Source: CAD feature listing. Evaluate the final solid. Frame: model axes, mm. Round coordinates to 2 decimals unless told otherwise and drop trailing zeros. Loops run counter-clockwise (first coordinate to the right, second up) from the corner with the lowest first, then second, coordinate; pieces in that order, holes last.
Item 1: Section query D-D on z = 1.5. Give the number of separate pieces and of enclosed holes in the cut face, then the cut area to 3 significant figures.
Item 2: Section query B-B on x = 19.05. Return loops of the section in (y, z) (3 decimals), then the cut area to 3 significant figures.
Item 3: Ray query, L1, parallel to Y at x = 25.4, z = -0.75; L2, parallel to X at y = 88, z = 0 (3 decimals); L3, parallel to Y at x = -24.5, z = 1.75. Return the intervals inside material, ascending.
Item 4: First-contact query: P1, Ø4.5, axis at x = -0.06, y = -40.99, coming from the -Z side. Flat tip, straight axial feed; report the tip coordinate or a pass-through.
Item 5: Section query C-C on y = -57.15. Return loops of the section in (x, z) (3 decimals), then the cut area to 3 significant figures.
Item 6: Section query A-A on y = 44.45. Return loops of the section in (x, z) (3 decimals).
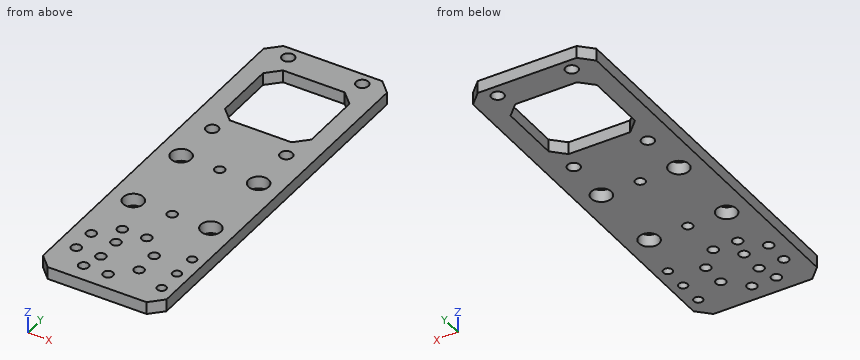
```python
from build123d import *

# Parameters (mm, degrees)
SKETCH1_W                       = 63.5
SKETCH1_H                       = 196.85
BOSS_EXTRUDE1_DEPTH             = 3.175
SKETCH2_R                       = 2.54
SKETCH2_R_2                     = 5.175
CUT_EXTRUDE1_DEPTH              = 7.35
SKETCH3_W                       = 44.45
SKETCH3_H                       = 44.45
CUT_EXTRUDE2_DEPTH              = 7.35
SKETCH4_R                       = 3.175
CUT_EXTRUDE3_DEPTH              = 7.35
CHAMFER1_SIZE                   = 6.35
SKETCH5_R                       = 2.286
CUT_EXTRUDE4_DEPTH              = 7.35
F_10_CLEARANCE_HOLE1_AT_2_COUNT = 2
F_10_CLEARANCE_HOLE1_AT_2_PITCH = 13.97
F_10_CLEARANCE_HOLE1_AT_3_COUNT = 2
F_10_CLEARANCE_HOLE1_AT_3_PITCH = 34.687510721
F_10_CLEARANCE_HOLE1_AT_4_COUNT = 2
F_10_CLEARANCE_HOLE1_AT_4_PITCH = 31.75
SKETCH9_R                       = 2.5527
CUT_EXTRUDE6_DEPTH              = 7.35


with BuildPart() as part:
    # Sketch1 → Boss-Extrude1 (new body, symmetric)
    with BuildSketch(Plane.XY):
        with Locations((0, 15.875)):
            Rectangle(SKETCH1_W, SKETCH1_H)
    extrude(amount=BOSS_EXTRUDE1_DEPTH, both=True)

    # Sketch2 → Cut-Extrude1 (cut, through all)
    with BuildSketch(Plane.XY.offset(3.175)):
        with Locations((0, 19.85)):
            Circle(SKETCH2_R)
        with Locations((0, -19.85)):
            Circle(SKETCH2_R)
        with Locations((-19.939, 19.939)):
            Circle(SKETCH2_R_2)
        with Locations((19.939, 19.939)):
            Circle(SKETCH2_R_2)
        with Locations((19.939, -19.939)):
            Circle(SKETCH2_R_2)
        with Locations((-19.939, -19.939)):
            Circle(SKETCH2_R_2)
    extrude(amount=-CUT_EXTRUDE1_DEPTH, mode=Mode.SUBTRACT)

    # Sketch3 → Cut-Extrude2 (cut, through all)
    with BuildSketch(Plane.XY.offset(3.175)):
        with Locations((0, 76.2)):
            Rectangle(SKETCH3_W, SKETCH3_H)
    extrude(amount=-CUT_EXTRUDE2_DEPTH, mode=Mode.SUBTRACT)

    # Sketch4 → Cut-Extrude3 (cut, through all)
    with BuildSketch(Plane.XY.offset(3.175)):
        with Locations((-19.05, 107.95)):
            Circle(SKETCH4_R)
        with Locations((19.05, 107.95)):
            Circle(SKETCH4_R)
        with Locations((19.05, 44.45)):
            Circle(SKETCH4_R)
        with Locations((-19.05, 44.45)):
            Circle(SKETCH4_R)
    extrude(amount=-CUT_EXTRUDE3_DEPTH, mode=Mode.SUBTRACT)

    # Chamfer1
    chamfer1_edges = [part.edges().sort_by_distance(p)[0] for p in [
        (22.225, 98.425, 0),
        (22.225, 53.975, 0),
        (-22.225, 53.975, 0),
        (-22.225, 98.425, 0),
        (31.75, -82.55, 0),
        (-31.75, -82.55, 0),
        (-31.75, 114.3, 0),
        (31.75, 114.3, 0),
    ]]
    chamfer(chamfer1_edges, length=CHAMFER1_SIZE)

    # Sketch5 → Cut-Extrude4 (cut, through all)
    with BuildSketch(Plane(origin=(0, 0, -3.175), x_dir=(-1, 0, 0), z_dir=(0, 0, -1))):
        with Locations((-25.4, -44.45)):
            Circle(SKETCH5_R)
        with Locations((-25.4, -57.15)):
            Circle(SKETCH5_R)
        with Locations((-25.4, -69.85)):
            Circle(SKETCH5_R)
    extrude(amount=-CUT_EXTRUDE4_DEPTH, mode=Mode.SUBTRACT)

    # Sketch8 → 10 Clearance Hole1 (revolve, cut)
    with BuildSketch(Plane(origin=(-22.514461018, -50.863820715, 3.175), x_dir=(0, -1, 0), z_dir=(1, 0, 0))):
        Polygon((0, 0), (0, 20.583816902), (2.5527, 19.05), (2.5527, 0), align=None)
    f_10_clearance_hole1 = revolve(axis=Axis((-22.514461018, -50.863820715, 9.525), (0, 0, -1)), mode=Mode.SUBTRACT)

    # 10 Clearance Hole1 at 2: 10 Clearance Hole1 ×2
    with Locations(*[Vector(0.707106781, 0.707106781, 0) * (i * F_10_CLEARANCE_HOLE1_AT_2_PITCH) for i in range(1, F_10_CLEARANCE_HOLE1_AT_2_COUNT)]):
        add(f_10_clearance_hole1, mode=Mode.SUBTRACT)

    # 10 Clearance Hole1 at 3: 10 Clearance Hole1 ×2
    with Locations(*[Vector(0.932004672, -0.362446261, 0) * (i * F_10_CLEARANCE_HOLE1_AT_3_PITCH) for i in range(1, F_10_CLEARANCE_HOLE1_AT_3_COUNT)]):
        add(f_10_clearance_hole1, mode=Mode.SUBTRACT)

    # 10 Clearance Hole1 at 4: 10 Clearance Hole1 ×2
    with Locations(*[Vector(0.707106781, -0.707106781, 0) * (i * F_10_CLEARANCE_HOLE1_AT_4_PITCH) for i in range(1, F_10_CLEARANCE_HOLE1_AT_4_COUNT)]):
        add(f_10_clearance_hole1, mode=Mode.SUBTRACT)

    # Mirror1: 10 Clearance Hole1 across plane
    add(f_10_clearance_hole1.mirror(Plane.ZY.offset(6.35)), mode=Mode.SUBTRACT)

    # Mirror1 copy 1 sketch → Mirror1 copy 1 (revolve, cut)
    with BuildSketch(Plane(origin=(-0.063820715, -40.985538982, 3.175), x_dir=(0, -1, 0), z_dir=(-1, 0, 0))):
        Polygon((0, 0), (0, -20.583816902), (2.5527, -19.05), (2.5527, 0), align=None)
    revolve(axis=Axis((-0.063820715, -40.985538982, 9.525), (0, 0, 1)), mode=Mode.SUBTRACT)

    # Mirror1 copy 2 sketch → Mirror1 copy 2 (revolve, cut)
    with BuildSketch(Plane(origin=(-22.514461018, -63.436179285, 3.175), x_dir=(0, -1, 0), z_dir=(-1, 0, 0))):
        Polygon((0, 0), (0, -20.583816902), (2.5527, -19.05), (2.5527, 0), align=None)
    revolve(axis=Axis((-22.514461018, -63.436179285, 9.525), (0, 0, 1)), mode=Mode.SUBTRACT)

    # Mirror1 copy 3 sketch → Mirror1 copy 3 (revolve, cut)
    with BuildSketch(Plane(origin=(-12.636179285, -73.314461018, 3.175), x_dir=(0, -1, 0), z_dir=(-1, 0, 0))):
        Polygon((0, 0), (0, -20.583816902), (2.5527, -19.05), (2.5527, 0), align=None)
    revolve(axis=Axis((-12.636179285, -73.314461018, 9.525), (0, 0, 1)), mode=Mode.SUBTRACT)

    # Sketch9 → Cut-Extrude6 (cut, through all)
    with BuildSketch(Plane.XY.offset(3.175)):
        with Locations((-9.814461018, -50.863820715)):
            Circle(SKETCH9_R)
        with Locations((-9.814461018, -63.436179285)):
            Circle(SKETCH9_R)
    extrude(amount=-CUT_EXTRUDE6_DEPTH, mode=Mode.SUBTRACT)


solid = part.part
```
Data:
1. separate pieces: 1
1. enclosed holes: 24
1. area: 9,770 mm2
2. outline: (-82.55, -3.175) - (-25.037, -3.175) - (-25.037, 3.175) - (-82.55, 3.175) - close; (-14.841, -3.175) - (14.841, -3.175) - (14.841, 3.175) - (-14.841, 3.175) - close; (25.037, -3.175) - (41.275, -3.175) - (41.275, 3.175) - (25.037, 3.175) - close; (47.625, -3.175) - (57.15, -3.175) - (57.15, 3.175) - (47.625, 3.175) - close; (95.25, -3.175) - (104.775, -3.175) - (104.775, 3.175) - (95.25, 3.175) - close; (111.125, -3.175) - (114.3, -3.175) - (114.3, 3.175) - (111.125, 3.175) - close
2. area: 798 mm2
3. L1: y = -82.55 to -72.14, -67.56 to -59.44, -54.86 to -46.74, -42.16 to 114.3
3. L2: x = -31.75 to -22.225, 22.225 to 31.75
3. L3: y = -82.55 to -65.04, -61.83 to -52.47, -49.26 to -22.38, -17.49 to 17.49, 22.38 to 114.3
4. P1: passes through
5. outline: (-31.75, -3.175) - (23.114, -3.175) - (23.114, 3.175) - (-31.75, 3.175) - close; (27.686, -3.175) - (31.75, -3.175) - (31.75, 3.175) - (27.686, 3.175) - close
5. area: 374 mm2
6. outline: (-31.75, -3.175) - (-22.225, -3.175) - (-22.225, 3.175) - (-31.75, 3.175) - close; (-15.875, -3.175) - (15.875, -3.175) - (15.875, 3.175) - (-15.875, 3.175) - close; (22.225, -3.175) - (31.75, -3.175) - (31.75, 3.175) - (22.225, 3.175) - close
